Can you work these out from the model? Positions are in its coordinate system, mm. A direction names the side the tool comes from. Round coordinates to 2 decimals unless told otherwise and drop trailing zeros. One line per item, written item: value.
```python
from build123d import *

# Parameters (mm, degrees)
CYLINDER158_R             = 1.6
CYLINDER158_DEPTH         = 9
CYLINDER159_R             = 1.6
CYLINDER159_DEPTH         = 9
CYLINDER156_R             = 1.6
CYLINDER156_DEPTH         = 9
CYLINDER157_R             = 1.6
CYLINDER157_DEPTH         = 9
BOX068_W                  = 59
BOX068_H                  = 20
BOX068_DEPTH              = 32
BOX068_PLACEMENT_ANGLE    = 3
BOX066_W                  = 128
BOX066_H                  = 3
BOX066_DEPTH              = 35
BOX066_PLACEMENT_ANGLE    = 3
CYLINDER147_W             = 52
CYLINDER147_H             = 3
CYLINDER147_ANGLE         = 180
CYLINDER147_ROLL_ANGLE    = 90
CYLINDER147_PITCH_ANGLE   = -3
BOX067_W                  = 128
BOX067_H                  = 3
BOX067_DEPTH              = 35
BOX067_PLACEMENT_ANGLE    = 3
CYLINDER148_W             = 52
CYLINDER148_H             = 3
CYLINDER148_ANGLE         = 180
CYLINDER148_ROLL_ANGLE    = 90
CYLINDER148_PITCH_ANGLE   = -3
BOX065_W                  = 7
BOX065_H                  = 30
BOX065_DEPTH              = 10
BOX065_PLACEMENT_ANGLE    = 3
CYLINDER144_W             = 49
CYLINDER144_H             = 53
CYLINDER144_ANGLE         = 180
CYLINDER143_W             = 52
CYLINDER143_H             = 53
CYLINDER143_ANGLE         = 180
CYLINDER146_W             = 48
CYLINDER146_H             = 2
CYLINDER146_ANGLE         = 180
CYLINDER145_W             = 52
CYLINDER145_H             = 2
CYLINDER145_ANGLE         = 180
FUSION121_PLACEMENT_ANGLE = 3
FILLET033_R               = 0.99


with BuildPart() as cylinder158:
    # Cylinder158 → Cylinder158 (new body)
    with BuildSketch(Plane(origin=(555, -5, 10), x_dir=(1, 0, 0), z_dir=(0, -1, 0))):
        Circle(CYLINDER158_R)
    extrude(amount=CYLINDER158_DEPTH)


with BuildPart() as fusion134:
    # Cylinder159 → Cylinder159 (new body)
    with BuildSketch(Plane(origin=(450, -5, 10), x_dir=(1, 0, 0), z_dir=(0, -1, 0))):
        Circle(CYLINDER159_R)
    extrude(amount=CYLINDER159_DEPTH)

    # Fusion134: union Cylinder158
    add(cylinder158.part)


with BuildPart() as fusion134_1:
    # Fusion134 placement: moved
    add(fusion134.part.moved(Location((9, 0, 0))))


with BuildPart() as cylinder156:
    # Cylinder156 → Cylinder156 (new body)
    with BuildSketch(Plane(origin=(555, -5, 10), x_dir=(1, 0, 0), z_dir=(0, -1, 0))):
        Circle(CYLINDER156_R)
    extrude(amount=CYLINDER156_DEPTH)


with BuildPart() as fusion136:
    # Cylinder157 → Cylinder157 (new body)
    with BuildSketch(Plane(origin=(450, -5, 10), x_dir=(1, 0, 0), z_dir=(0, -1, 0))):
        Circle(CYLINDER157_R)
    extrude(amount=CYLINDER157_DEPTH)

    # Fusion133: union Cylinder156
    add(cylinder156.part)


with BuildPart() as fusion136_1:
    # Fusion133 placement: moved
    add(fusion136.part.moved(Location((-9, 0, 0))))

    # Fusion136: union Fusion134
    add(fusion134_1.part)


with BuildPart() as cube047:
    # Box068 → Box068 (new body)
    with BuildSketch(Plane.XY):
        with Locations((29.5, 10)):
            Rectangle(BOX068_W, BOX068_H)
    extrude(amount=BOX068_DEPTH)


with BuildPart() as cube047_1:
    # Box068 placement: moved
    add(cube047.part.moved(Location((473, -20, -36))).rotate(Axis((473, -20, -36), (0, -1, 0)), BOX068_PLACEMENT_ANGLE))


with BuildPart() as cube045:
    # Box066 → Box066 (new body)
    with BuildSketch(Plane.XY):
        with Locations((64, 1.5)):
            Rectangle(BOX066_W, BOX066_H)
    extrude(amount=BOX066_DEPTH)


with BuildPart() as cube045_1:
    # Box066 placement: moved
    add(cube045.part.moved(Location((382, -9, -40.8))).rotate(Axis((382, -9, -40.8), (0, -1, 0)), BOX066_PLACEMENT_ANGLE))


with BuildPart() as cut079:
    # Cylinder147 → Cylinder147 (revolve)
    with BuildSketch(Plane.XZ):
        with Locations((26, 1.5)):
            Rectangle(CYLINDER147_W, CYLINDER147_H)
    revolve(axis=Axis((0, 0, 0), (0, 0, 1)), revolution_arc=CYLINDER147_ANGLE)


with BuildPart() as cut079_1:
    # Cylinder147 roll: moved
    add(cut079.part.rotate(Axis((0, 0, 0), (1, 0, 0)), CYLINDER147_ROLL_ANGLE))


with BuildPart() as cut079_2:
    # Cylinder147 pitch: moved
    add(cut079_1.part.rotate(Axis((0, 0, 0), (0, 1, 0)), CYLINDER147_PITCH_ANGLE))


with BuildPart() as cut079_3:
    # Cylinder147 placement: moved
    add(cut079_2.part.moved(Location((448.581401, -6, -35.39126))))

    # Cut079: cut Cube045
    add(cube045_1.part, mode=Mode.SUBTRACT)


with BuildPart() as cut079_4:
    # Cut079 placement: moved
    add(cut079_3.part.moved(Location((0.48, 0, -0.5))))


with BuildPart() as cube046:
    # Box067 → Box067 (new body)
    with BuildSketch(Plane.XY):
        with Locations((64, 1.5)):
            Rectangle(BOX067_W, BOX067_H)
    extrude(amount=BOX067_DEPTH)


with BuildPart() as cube046_1:
    # Box067 placement: moved
    add(cube046.part.moved(Location((382, -9, -40.8))).rotate(Axis((382, -9, -40.8), (0, -1, 0)), BOX067_PLACEMENT_ANGLE))


with BuildPart() as cut080:
    # Cylinder148 → Cylinder148 (revolve)
    with BuildSketch(Plane.XZ):
        with Locations((26, 1.5)):
            Rectangle(CYLINDER148_W, CYLINDER148_H)
    revolve(axis=Axis((0, 0, 0), (0, 0, 1)), revolution_arc=CYLINDER148_ANGLE)


with BuildPart() as cut080_1:
    # Cylinder148 roll: moved
    add(cut080.part.rotate(Axis((0, 0, 0), (1, 0, 0)), CYLINDER148_ROLL_ANGLE))


with BuildPart() as cut080_2:
    # Cylinder148 pitch: moved
    add(cut080_1.part.rotate(Axis((0, 0, 0), (0, 1, 0)), CYLINDER148_PITCH_ANGLE))


with BuildPart() as cut080_3:
    # Cylinder148 placement: moved
    add(cut080_2.part.moved(Location((448.581401, -6, -35.39126))))

    # Cut080: cut Cube046
    add(cube046_1.part, mode=Mode.SUBTRACT)


with BuildPart() as cut080_4:
    # Cut080 placement: moved
    add(cut080_3.part.moved(Location((105.48, 0, 5))))


with BuildPart() as cube044:
    # Box065 → Box065 (new body)
    with BuildSketch(Plane.XY):
        with Locations((3.5, 15)):
            Rectangle(BOX065_W, BOX065_H)
    extrude(amount=BOX065_DEPTH)


with BuildPart() as cube044_1:
    # Box065 placement: moved
    add(cube044.part.moved(Location((498, -39, -32.8))).rotate(Axis((498, -39, -32.8), (0, -1, 0)), BOX065_PLACEMENT_ANGLE))


with BuildPart() as cylinder144:
    # Cylinder144 → Cylinder144 (revolve)
    with BuildSketch(Plane(origin=(450, -9, -42), x_dir=(1, 0, 0), z_dir=(0, 0, -1))):
        with Locations((24.5, 26.5)):
            Rectangle(CYLINDER144_W, CYLINDER144_H)
    revolve(axis=Axis((450, -9, -42), (0, -1, 0)), revolution_arc=CYLINDER144_ANGLE)


with BuildPart() as cylinder143:
    # Cylinder143 → Cylinder143 (revolve)
    with BuildSketch(Plane(origin=(450, -9, -42), x_dir=(1, 0, 0), z_dir=(0, 0, -1))):
        with Locations((26, 26.5)):
            Rectangle(CYLINDER143_W, CYLINDER143_H)
    revolve(axis=Axis((450, -9, -42), (0, -1, 0)), revolution_arc=CYLINDER143_ANGLE)


with BuildPart() as cut077:
    # Cut077 base: copy of Cylinder143
    add(cylinder143.part)

    # Cut077: cut Cylinder144
    add(cylinder144.part, mode=Mode.SUBTRACT)


with BuildPart() as cut077_1:
    # Cut077 placement: moved
    add(cut077.part.moved(Location((0, 0, 10))))


with BuildPart() as cylinder146:
    # Cylinder146 → Cylinder146 (revolve)
    with BuildSketch(Plane(origin=(450, -12, -42), x_dir=(1, 0, 0), z_dir=(0, 0, -1))):
        with Locations((24, 1)):
            Rectangle(CYLINDER146_W, CYLINDER146_H)
    revolve(axis=Axis((450, -12, -42), (0, -1, 0)), revolution_arc=CYLINDER146_ANGLE)


with BuildPart() as cylinder145:
    # Cylinder145 → Cylinder145 (revolve)
    with BuildSketch(Plane(origin=(450, -12, -42), x_dir=(1, 0, 0), z_dir=(0, 0, -1))):
        with Locations((26, 1)):
            Rectangle(CYLINDER145_W, CYLINDER145_H)
    revolve(axis=Axis((450, -12, -42), (0, -1, 0)), revolution_arc=CYLINDER145_ANGLE)


with BuildPart() as fusion120:
    # Cut078 base: copy of Cylinder145
    add(cylinder145.part)

    # Cut078: cut Cylinder146
    add(cylinder146.part, mode=Mode.SUBTRACT)


with BuildPart() as fusion120_1:
    # Cut078 placement: moved
    add(fusion120.part.moved(Location((0, -48, 10))))

    # Fusion120: union Cut077
    add(cut077_1.part)


with BuildPart() as cut075:
    # Cut075 base: copy of Cylinder143
    add(cylinder143.part)

    # Cut075: cut Cylinder144
    add(cylinder144.part, mode=Mode.SUBTRACT)


with BuildPart() as cut075_1:
    # Cut075 placement: moved
    add(cut075.part.moved(Location((0, 0, 10))))


with BuildPart() as fender_lh:
    # Cut076 base: copy of Cylinder145
    add(cylinder145.part)

    # Cut076: cut Cylinder146
    add(cylinder146.part, mode=Mode.SUBTRACT)


with BuildPart() as fender_lh_1:
    # Cut076 placement: moved
    add(fender_lh.part.moved(Location((0, -48, 10))))

    # Fusion119: union Cut075
    add(cut075_1.part)


with BuildPart() as fender_lh_2:
    # Fusion119 placement: moved
    add(fender_lh_1.part.moved(Location((105, 0, 0))))

    # Fusion121: union Fusion120
    add(fusion120_1.part)


with BuildPart() as fender_lh_3:
    # Fusion121 placement: moved
    add(fender_lh_2.part.moved(Location((-2, 0, -27))).rotate(Axis((-2, 0, -27), (0, -1, 0)), FUSION121_PLACEMENT_ANGLE))

    # Fusion122: union Cube044
    add(cube044_1.part)


with BuildPart() as fender_lh_4:
    # Fusion122 placement: moved
    add(fender_lh_3.part.moved(Location((0, 3, 0))))

    # Fusion123: union Cut079, Cut080
    add(cut079_4.part)
    add(cut080_4.part)

    # Cut081: cut Cube047
    add(cube047_1.part, mode=Mode.SUBTRACT)

    # Fillet033
    fillet033_edges = [fender_lh_4.edges().sort_by_distance(p)[0] for p in [
        (551.349681, -57, 19.023158),
        (446.493579, -57, 13.527882),
    ]]
    fillet(fillet033_edges, radius=FILLET033_R)


with BuildPart() as fender_lh_5:
    # Fillet033 placement: moved
    add(fender_lh_4.part.moved(Location((0, -3, 2))))

    # Cut084: cut Fusion136
    add(fusion136_1.part, mode=Mode.SUBTRACT)


solid = fender_lh_5.part
```
Q1. On a 3-axis mill with a long thin cutter (end or side, diameter ignored), from which of +Z, -Z, +X, -X, +Y, -Y can I reach the whole of each face in a straight line? I mean faces 5 (the face through (442, -9, 4)), 6 (the face through (487.893, -15.902, -1.176)). Say none if no direction works.
Answers below:
face 5: +Z, -Z, +X, -X, +Y
face 6: -Z, +Y
Q2. Please list where these lines run through material, in increasing order: line 1 along X through (y, z) = (-24, 11.5); line 2 along X through (y, z) = (-46, -26); line 3 along X through (y, z) = (-10.55, 10).
Answers below:
line 1: 422.84 to 429.45, 468.67 to 475.28, 519.99 to 524.8, 583.03 to 587.84
line 2: 397.59 to 400.62, 497.5 to 500.53, 501.95 to 504.95
line 3: 420.42 to 439.4, 442.6 to 457.4, 460.6 to 477.69, 518.32 to 544.4, 547.6 to 562.4, 565.6 to 589.51
Q3. I want a section at B-B on z = -13.5. Give the number of separate pieces and of enclosed holes in the cut face, plus the area to 3 significant figures.
Answers below:
separate pieces: 4
enclosed holes: 0
area: 598 mm^2
Q4. Will these pins go through, and if not, where does the flat tip stop? pin 1 Ø9 at (x, z) = (555.5, 10) entering from -Y; pin 2 Ø2 at (x, y) = (560.5, -41.5) entering from +Z; pin 3 Ø1 at (x, y) = (426.5, -33) entering from +Z; pin 4 Ø1.9 at (x, z) = (459, 10) entering from +Y.
Answers below:
pin 1: y = -12
pin 2: z = 23.79
pin 3: z = 13.68
pin 4: through
Q5. We'd pull the mould along Y, two halves only. Please class faces 1 (the face through (504, -23, -16)), 2 (the face through (447.57, -34.355, 15.572)), 3 (the face through (552.46, -61.01, 20.07)), 4 (the face through (552.426, -34.355, 21.068)): released by +Y, released by -Y, zero draft, split by the parting line, or undercut.
Answers below:
face 1: released by +Y
face 2: undercut
face 3: zero draft
face 4: undercut
